Input: part model. Units: mm. Frame: model coordinates. Face numbers are marked on the shaded views. A direction names the side the tool comes from. Coordinates: 2 decimals unless noted, no trailing zeros. Loops run counter-clockwise (first coordinate to the right, second up) from the corner with the lowest first, then second, coordinate; pieces in that order, holes last. Notation, with made-up numbers: M 3.5,-30.75 L 21.5,-30.75 A23 ccw 21.5,3.25 Z; hole C -32.75,5 d10. An arc over 180 degrees is marked long. Use a Markdown table: item, result. Add a question column.
1. Section A-A on y = 0. Output: boundary loops of the cut face in (x, z) (3 decimals), then the cut area to 3 significant figures.
2. Section B-B on z = 0. Output: boundary loops of the cut face in (x, y) (3 decimals).
3. Section C-C on y = 2.75. Output: boundary loops of the cut face in (x, z).
4. Pin query (flat end, axial travel): pin 1 (3 mm diameter, centred on x = 7, z = 4, fed in from +Y); pin 2 (3 mm diameter, centred on x = 4, y = 2.5, fed in from +Z); pin 3 (2.5 mm diameter, centred on x = 4.5, y = 0, fed in from -Z); pin 4 (5 mm diameter, centred on y = -4.5, z = 4.5, fed in from -X). Return the tip coordinate at first contact, or that it passes through.
5. Set-up query: the marked faces 4 and 5. Return all of +Z, -Z, +X, -X, +Y, -Y with unobstructed straight access to the full face (end or side cutting, diameter ignored); none if empty.
6. Line query: L1, parallel to X at y = 0.25, z = -5.5; L2, parallel to Z at x = 2.5, y = 0 (3 decimals); L3, parallel to X at y = 0, z = -3.55. Output: solid intervals per line, ascending. Write a range as [from, to].
7. Section D-D on x = 5.25. Output: boundary loops of the cut face in (y, z) (3 decimals).
8. Draft query along X for the marked faces 1, 2 and 3. Return one class per face: +X half, -X half, draft (parallel to the pull), parting line (faces both ways), or undercut.
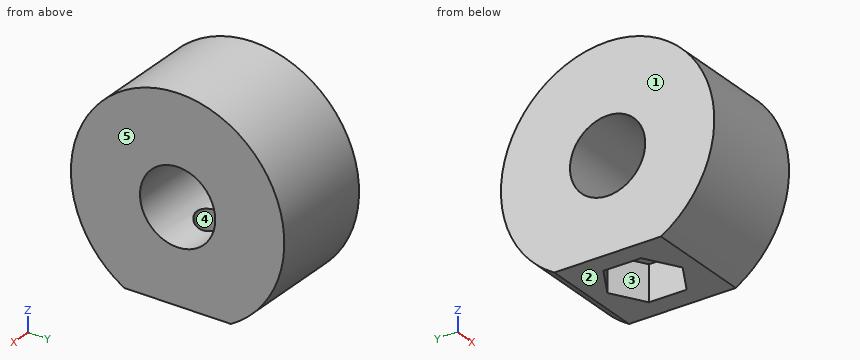
```python
from build123d import *

# Parameters (mm, degrees)
F0_R     = 3.175
F1_DEPTH = 9
F3_DEPTH = 3
F4_R     = 1.5
F5_DEPTH = 6


with BuildPart() as f1:
    # F0 (on Right) → F1 (new body)
    with BuildSketch(Plane.YZ):
        with BuildLine():
            ThreePointArc((4.5, -7.794229), (0, 9), (-4.5, -7.794229))
            Line((-4.5, -7.794229), (4.5, -7.794229))
        make_face()
        Circle(F0_R, mode=Mode.SUBTRACT)
    extrude(amount=F1_DEPTH)

    # F2 (on face) → F3 (cut)
    with BuildSketch(Plane(origin=(0, 0, -7.794229), x_dir=(1, 0, 0), z_dir=(0, 0, -1))):
        Polygon((1.75, 1.587713), (1.75, -1.587713), (4.5, -3.175426), (7.25, -1.587713), (7.25, 1.587713), (4.5, 3.175426), align=None)
    extrude(amount=-F3_DEPTH, mode=Mode.SUBTRACT)

    # F4 (on face) → F5 (cut)
    with BuildSketch(Plane(origin=(0, 0, -7.794229), x_dir=(1, 0, 0), z_dir=(0, 0, -1))):
        with Locations((4.5, 0)):
            Circle(F4_R)
    extrude(amount=-F5_DEPTH, mode=Mode.SUBTRACT)


solid = f1.part
```
Answers below:
| question | item | result |
|---|---|---|
| 1 | outline | M 0,-7.794 L 1.75,-7.794 L 1.75,-4.794 L 3,-4.794 L 3,-3.175 L 0,-3.175 Z; M 0,3.175 L 9,3.175 L 9,9 L 0,9 Z; M 6,-4.794 L 7.25,-4.794 L 7.25,-7.794 L 9,-7.794 L 9,-3.175 L 6,-3.175 Z |
| 1 | area | 72.6 mm² |
| 2 | outline | M 0,-9 L 9,-9 L 9,-3.175 L 0,-3.175 Z; M 0,3.175 L 9,3.175 L 9,9 L 0,9 Z |
| 3 | outline | M 0,-7.79 L 3.76,-7.79 L 3.76,-4.79 L 5.24,-4.79 L 5.24,-7.79 L 9,-7.79 L 9,-1.59 L 0,-1.59 Z; M 0,1.59 L 9,1.59 L 9,8.57 L 0,8.57 Z |
| 4 | pin 1 | stops at y = 8.65 |
| 4 | pin 2 | stops at z = 8.94 |
| 4 | pin 3 | stops at z = 2.92 |
| 4 | pin 4 | stops at x = 0 |
| 5 | face 4 | -Z |
| 5 | face 5 | +Z, -Z, +X, +Y, -Y |
| 6 | L1 | x = [0, 1.75], [7.25, 9] |
| 6 | L2 | z = [-4.794, -3.175], [3.175, 9] |
| 6 | L3 | x = [0, 3], [6, 9] |
| 7 | outline | M -4.5,-7.794 L -2.742,-7.794 L -2.742,-4.794 L -1.299,-4.794 L -1.299,-2.897 A3.175 cw long 1.299,-2.897 L 1.299,-4.794 L 2.742,-4.794 L 2.742,-7.794 L 4.5,-7.794 A9 ccw long Z |
| 8 | face 1 | -X half |
| 8 | face 2 | draft |
| 8 | face 3 | undercut |
